Read the model definition and answer for the solid it produces. Units are mm, in the model's axes. A direction names the side the tool comes from. Give positions to 0.01 mm unless a question says otherwise; leave off trailing zeros. Order: outer loops, then holes, each group sorted by start corner. A loop starts at its lowest first (then second) coordinate and runs counter-clockwise, first axis right, second up. Notation, with made-up numbers: (-16, 25) - (-5, 25) arc R21 cw to (-5, 58) - close; hole circle Ø10 at (41.25, 12.5). An arc over 180 degrees is marked (long way). Answer as CSV lines item,"result". Start each with the question number.
from build123d import *

# Parameters (mm, degrees)
SKETCH1_W           = 9.525
SKETCH1_H           = 19.05
BOSS_EXTRUDE1_DEPTH = 9.525
SKETCH2_R           = 1.28905
CUT_EXTRUDE1_DEPTH  = 12.7
SKETCH4_R           = 2.0193
CUT_EXTRUDE2_DEPTH  = 17.497783942


with BuildPart() as part:
    # Sketch1 → Boss-Extrude1 (new body)
    with BuildSketch(Plane.XY):
        Rectangle(SKETCH1_W, SKETCH1_H)
    extrude(amount=BOSS_EXTRUDE1_DEPTH)

    # Sketch2 → Cut-Extrude1 (cut)
    with BuildSketch(Plane.XZ.offset(9.525)):
        with Locations(Location((0, 4.7625, 0), (0, 0, 270))):
            Circle(SKETCH2_R)
    extrude(amount=-CUT_EXTRUDE1_DEPTH, mode=Mode.SUBTRACT)

    # Sketch4 → Cut-Extrude2 (cut, through all)
    with BuildSketch(Plane.ZY.offset(4.7625)):
        with Locations(Location((4.7625, 6.35, 0), (0, 0, 270))):
            Circle(SKETCH4_R)
    extrude(amount=-CUT_EXTRUDE2_DEPTH, mode=Mode.SUBTRACT)


solid = part.part
(1) Section D-D, the plane y = -5.5 is taken. Write down the section's boundary in (x, z) (1 decimal), and give its area (3 significant figures).
(2) Determine the mould class of faces 3 (the flat face through (0, 3.175, 5)), 4 (the flat face through (-4.762, 0, 5)), 5 (the flat face through (0, 0, 0)) for opening direction X: released by +X, released by -X, zero draft, split by the parting line, or undercut.
(3) Straight lines are drawn through the part: line 1 (Z direction, x = 2, y = 6.35) (3 decimals); line 2 (X direction, y = -6.75, z = 4.75); line 3 (Y direction, x = -3.5, z = 5) (3 decimals). For each, find the intervals that lie inside material, in ascending order. Write a range as [from, to].
(4) Section A-A, the plane y = 6.35 is taken. Write down the section's boundary in (x, z) (1 decimal).
(5) Which of the six approach directions +Z, -Z, +X, -X, +Y, -Y give full straight-line access (tool end or side, diameter ignored) to faces 1 (the flat face through (0, 9.525, 5)), 2 (the cylindrical face through (0.06, -3.26, 6.05))?
(6) Section C-C, the plane z = 6.5 is taken. Write down the section's boundary in (x, y) (1 decimal), and give its area (3 significant figures).
(7) A flat-ended cylindrical pin translates along its axis: pin 1 Ø1.3 at (x, z) = (0, 5) entering from -Y (3 decimals). Find the tip coordinate at first contact, or state that the pin passes through.
Checks:
1,outline,"(-4.8, 0) - (4.8, 0) - (4.8, 9.5) - (-4.8, 9.5) - close; hole circle Ø2.6 at (0, 4.8)"
1,area,"85.5 mm²"
2,face 3,"undercut"
2,face 4,"released by -X"
2,face 5,"zero draft"
3,line 1,"z = [0, 2.743], [6.782, 9.525]"
3,line 2,"x = [-4.76, -1.29], [1.29, 4.76]"
3,line 3,"y = [-9.525, 4.345], [8.355, 9.525]"
4,outline,"(-4.8, 0) - (4.8, 0) - (4.8, 2.7) - (-4.8, 2.7) - close; (-4.8, 6.8) - (4.8, 6.8) - (4.8, 9.5) - (-4.8, 9.5) - close"
5,face 1,"+Z, -Z, +X, -X, +Y"
5,face 2,"-Y"
6,outline,"(-4.8, -9.5) - (4.8, -9.5) - (4.8, 5.3) - (-4.8, 5.3) - close; (-4.8, 7.4) - (4.8, 7.4) - (4.8, 9.5) - (-4.8, 9.5) - close"
6,area,"162 mm²"
7,pin 1,"stops at y = 3.175"
